from build123d import *

# Parameters (mm, degrees)
SKETCH1_R           = 20
BOSS_EXTRUDE1_DEPTH = 2
CUT_EXTRUDE10_DEPTH = 29.354893758
CIRPATTERN1_DEPTH   = 2
SKETCH5_R           = 0.76
CUT_EXTRUDE11_DEPTH = 28.141520821
SCALE1_SCALE        = 1.5
SCALE2_SCALE        = 0.93


# Read off the part's stored shape, not the designer's step: CirPattern1
with BuildPart() as part:
    # Sketch1 → Boss-Extrude1 (new body)
    with BuildSketch(Plane(origin=(0, 0, 0), x_dir=(1, 0, 0), z_dir=(0, 1, 0))):
        with Locations(Location((0, 0, 0), (0, 0, 270))):
            Circle(SKETCH1_R)
    extrude(amount=BOSS_EXTRUDE1_DEPTH)

    # Sketch3 → Cut-Extrude10 (cut, through all)
    with BuildSketch(Plane(origin=(0, 2, 0), x_dir=(1, 0, 0), z_dir=(0, 1, 0))):
        with BuildLine():
            Line((-0.11374729, 19.999676536), (2.525531299, 21.841438752))
            Line((2.525531299, 21.841438752), (8.448237607, 18.128079913))
            add(Edge.make_bspline(
                [(0.314716636, 11.921594207), (-1.061906761, 18.280624108), (8.448237607, 18.128079913)],
                knots=[0, 0, 0, 1, 1, 1], degree=2))
            add(Edge.make_bspline(
                [(-0.11374729, 19.999676536), (-3.476973379, 16.23883842), (0.314716636, 11.921594207)],
                knots=[0, 0, 0, 1, 1, 1], degree=2))
        make_face()
    extrude(amount=-CUT_EXTRUDE10_DEPTH, mode=Mode.SUBTRACT)

    # CirPattern1 outline → CirPattern1 (cut)
    with BuildSketch(Plane(origin=(0, 0, 0), x_dir=(1, 0, 0), z_dir=(0, 1, 0))):
        with BuildLine():
            add(Edge.make_bspline(
                [(-7.207557435, 17.244057808), (-7.782239787, 13.703261178), (-3.697405485, 11.367556407)],
                knots=[0.181076354, 0.181076354, 0.181076354, 1, 1, 1], degree=2))
            add(Edge.make_bspline(
                [(-3.697405485, 11.367556407), (-6.402099222, 15.840148745), (-1.097148713, 18.619435028)],
                knots=[0, 0, 0, 0.803340706, 0.803340706, 0.803340706], degree=2))
            add(Edge.make_bspline(
                [(-0.11374729, 19.999676536), (-0.722748007, 19.318677683), (-1.097148713, 18.619435028)],
                knots=[0, 0, 0, 0.181076354, 0.181076354, 0.181076354], degree=2))
            ThreePointArc((-0.11374729, 19.999676536), (-4.271024547, -19.538637345), (8.448237607, 18.128079913))
            add(Edge.make_bspline(
                [(5.128765463, 17.936244047), (6.577979327, 18.158079147), (8.448237607, 18.128079913)],
                knots=[0.803340706, 0.803340706, 0.803340706, 1, 1, 1], degree=2))
            add(Edge.make_bspline(
                [(5.128765463, 17.936244047), (2.500458036, 15.495035196), (4.289346694, 11.142878787)],
                knots=[0.181076354, 0.181076354, 0.181076354, 1, 1, 1], degree=2))
            add(Edge.make_bspline(
                [(4.289346694, 11.142878787), (4.902086374, 16.33363986), (10.795510687, 15.268519209)],
                knots=[0, 0, 0, 0.803340706, 0.803340706, 0.803340706], degree=2))
            add(Edge.make_bspline(
                [(10.795510687, 15.268519209), (7.516952988, 13.812991814), (7.795771849, 9.115796046)],
                knots=[0.181076354, 0.181076354, 0.181076354, 1, 1, 1], degree=2))
            add(Edge.make_bspline(
                [(7.795771849, 9.115796046), (10.060748967, 13.826351118), (15.289007186, 10.905349896)],
                knots=[0, 0, 0, 0.803340706, 0.803340706, 0.803340706], degree=2))
            add(Edge.make_bspline(
                [(15.289007186, 10.905349896), (11.715481814, 10.593232934), (10.454016527, 6.060011853)],
                knots=[0.181076354, 0.181076354, 0.181076354, 1, 1, 1], degree=2))
            add(Edge.make_bspline(
                [(10.454016527, 6.060011853), (14.125785669, 9.779899189), (18.12231489, 5.319553202)],
                knots=[0, 0, 0, 0.803340706, 0.803340706, 0.803340706], degree=2))
            add(Edge.make_bspline(
                [(18.12231489, 5.319553202), (14.641068768, 6.18466939), (11.97601867, 2.306667841)],
                knots=[0.181076354, 0.181076354, 0.181076354, 1, 1, 1], degree=2))
            add(Edge.make_bspline(
                [(11.97601867, 2.306667841), (16.656686676, 4.632779929), (18.988400946, -0.883563127)],
                knots=[0, 0, 0, 0.803340706, 0.803340706, 0.803340706], degree=2))
            add(Edge.make_bspline(
                [(18.988400946, -0.883563127), (15.976681108, 1.065037449), (12.196845731, -1.737502929)],
                knots=[0.181076354, 0.181076354, 0.181076354, 1, 1, 1], degree=2))
            add(Edge.make_bspline(
                [(12.196845731, -1.737502929), (17.379189594, -1.057236426), (17.793411491, -7.031795185)],
                knots=[0, 0, 0, 0.803340706, 0.803340706, 0.803340706], degree=2))
            add(Edge.make_bspline(
                [(17.793411491, -7.031795185), (15.577584513, -4.210871331), (11.09256767, -5.6342518)],
                knots=[0.181076354, 0.181076354, 0.181076354, 1, 1, 1], degree=2))
            add(Edge.make_bspline(
                [(11.09256767, -5.6342518), (16.215000021, -6.673548315), (14.666842175, -12.458886631)],
                knots=[0, 0, 0, 0.803340706, 0.803340706, 0.803340706], degree=2))
            add(Edge.make_bspline(
                [(14.666842175, -12.458886631), (13.487027293, -9.071330369), (8.782850151, -8.961305569)],
                knots=[0.181076354, 0.181076354, 0.181076354, 1, 1, 1], degree=2))
            add(Edge.make_bspline(
                [(8.782850151, -8.961305569), (13.29027596, -11.607541197), (9.947505297, -16.576727895)],
                knots=[0, 0, 0, 0.803340706, 0.803340706, 0.803340706], degree=2))
            add(Edge.make_bspline(
                [(9.947505297, -16.576727895), (9.93155376, -12.989633509), (5.517986904, -11.358126335)],
                knots=[0.181076354, 0.181076354, 0.181076354, 1, 1, 1], degree=2))
            add(Edge.make_bspline(
                [(5.517986904, -11.358126335), (8.921956647, -15.324540386), (4.146814235, -18.939086981)],
                knots=[0, 0, 0, 0.803340706, 0.803340706, 0.803340706], degree=2))
            add(Edge.make_bspline(
                [(4.146814235, -18.939086981), (5.296454639, -15.541171808), (1.651776524, -12.564981378)],
                knots=[0.181076354, 0.181076354, 0.181076354, 1, 1, 1], degree=2))
            add(Edge.make_bspline(
                [(1.651776524, -12.564981378), (3.58341726, -17.421751343), (-2.106636126, -19.289965628)],
                knots=[0, 0, 0, 0.803340706, 0.803340706, 0.803340706], degree=2))
            add(Edge.make_bspline(
                [(-2.106636126, -19.289965628), (0.084014843, -16.4494465), (-2.396817106, -12.451089227)],
                knots=[0.181076354, 0.181076354, 0.181076354, 1, 1, 1], degree=2))
            add(Edge.make_bspline(
                [(-2.396817106, -12.451089227), (-2.146828623, -17.671908721), (-8.135187408, -17.591340689)],
                knots=[0, 0, 0, 0.803340706, 0.803340706, 0.803340706], degree=2))
            add(Edge.make_bspline(
                [(-8.135187408, -17.591340689), (-5.140916898, -15.616031929), (-6.189066045, -11.028791865)],
                knots=[0.181076354, 0.181076354, 0.181076354, 1, 1, 1], degree=2))
            add(Edge.make_bspline(
                [(-6.189066045, -11.028791865), (-7.647819946, -16.047904086), (-13.285552537, -14.027284533)],
                knots=[0, 0, 0, 0.803340706, 0.803340706, 0.803340706], degree=2))
            add(Edge.make_bspline(
                [(-13.285552537, -14.027284533), (-9.812138156, -13.131241495), (-9.314021278, -8.452217279)],
                knots=[0.181076354, 0.181076354, 0.181076354, 1, 1, 1], degree=2))
            add(Edge.make_bspline(
                [(-9.314021278, -8.452217279), (-12.323438943, -12.725723538), (-16.999609535, -8.984017946)],
                knots=[0, 0, 0, 0.803340706, 0.803340706, 0.803340706], degree=2))
            add(Edge.make_bspline(
                [(-16.999609535, -8.984017946), (-13.423449627, -9.264340798), (-11.433045416, -5.000577306)],
                knots=[0.181076354, 0.181076354, 0.181076354, 1, 1, 1], degree=2))
            add(Edge.make_bspline(
                [(-11.433045416, -5.000577306), (-15.667009745, -8.06537689), (-18.874882696, -3.008057118)],
                knots=[0, 0, 0, 0.803340706, 0.803340706, 0.803340706], degree=2))
            add(Edge.make_bspline(
                [(-18.874882696, -3.008057118), (-15.583509678, -4.434368529), (-12.316509314, -1.047910694)],
                knots=[0.181076354, 0.181076354, 0.181076354, 1, 1, 1], degree=2))
            add(Edge.make_bspline(
                [(-12.316509314, -1.047910694), (-17.316204575, -2.571885013), (-18.708157077, 3.253009868)],
                knots=[0, 0, 0, 0.803340706, 0.803340706, 0.803340706], degree=2))
            add(Edge.make_bspline(
                [(-18.708157077, 3.253009868), (-16.058242285, 0.835272872), (-11.868675951, 2.977449797)],
                knots=[0.181076354, 0.181076354, 0.181076354, 1, 1, 1], degree=2))
            add(Edge.make_bspline(
                [(-11.868675951, 2.977449797), (-17.092307584, 3.159447008), (-16.517499984, 9.120699256)],
                knots=[0, 0, 0, 0.803340706, 0.803340706, 0.803340706], degree=2))
            add(Edge.make_bspline(
                [(-16.517499984, 9.120699256), (-14.796202804, 5.973535993), (-10.13807502, 6.639293898)],
                knots=[0.181076354, 0.181076354, 0.181076354, 1, 1, 1], degree=2))
            add(Edge.make_bspline(
                [(-10.13807502, 6.639293898), (-15.019581485, 8.507540416), (-12.540303105, 13.959155852)],
                knots=[0, 0, 0, 0.803340706, 0.803340706, 0.803340706], degree=2))
            add(Edge.make_bspline(
                [(-12.540303105, 13.959155852), (-11.934152795, 10.423610295), (-7.312243985, 9.540803981)],
                knots=[0.181076354, 0.181076354, 0.181076354, 1, 1, 1], degree=2))
            add(Edge.make_bspline(
                [(-7.312243985, 9.540803981), (-11.322638312, 12.892846308), (-7.207557435, 17.244057808)],
                knots=[0, 0, 0, 0.803340706, 0.803340706, 0.803340706], degree=2))
        make_face()
    extrude(amount=CIRPATTERN1_DEPTH, mode=Mode.SUBTRACT)

    # Sketch5 → Cut-Extrude11 (cut, through all)
    with BuildSketch(Plane(origin=(0, 2, 0), x_dir=(1, 0, 0), z_dir=(0, 1, 0))):
        with Locations(Location((0, 0, 0), (0, 0, 270))):
            Circle(SKETCH5_R)
    extrude(amount=-CUT_EXTRUDE11_DEPTH, mode=Mode.SUBTRACT)


with BuildPart() as part_1:
    # Scale1: scaled about (-0.031329983, 0.999999987, 0.377918145)
    add(part.part.scale(SCALE1_SCALE).moved(Location((0.015664991, -0.499999994, -0.188959072))))


with BuildPart() as part_2:
    # Scale2: scaled about (-0.031329983, 0.999999987, 0.377918146)
    add(part_1.part.scale(SCALE2_SCALE).moved(Location((-0.002193099, 0.069999999, 0.02645427))))


solid = part_2.part
Geometry check sheet. Reference: the model listing, model coordinates, mm. Give positions to 0.01 mm unless a question says otherwise; leave off trailing zeros. One line per question, with ' | ' between items.
1. Scan lines: line 1 along Z through (x, y) = (22, 1.4); line 2 along Z through (x, y) = (-22.5, 2.3); line 3 along Z through (x, y) = (16.5, 1.05). Record each from-to range of solid material in increasing order. Write a range as from..to.
Ans:
line 1: -10.27..-7.6, -4.05..0.03, 3.16..7.51 | line 2: -12.04..-7.79, -2.96..1.11, 4.54..7.88, 12.38..13.26 | line 3: -16.92..-12.69, -10.13..7.42, 7.96..13.11
2. Cross-section at A-A (z = -20.5). Count the separate pieces of the cut face and the enclosed holes in it, plus the area to 3 significant figures.
Ans:
separate pieces: 4 | enclosed holes: 0 | area: 47.9 mm2
3. Gauge pin test, flat ends, axial feed: pin 1 (1 mm diameter, centred on y = 1, z = 12, fed in from +X); pin 2 (1.5 mm diameter, centred on y = 1.5, z = 13.5, fed in from -X). Record the tip position at first contact, or that the pin passes through.
Ans:
pin 1: x = 20.86 | pin 2: x = -23.23
4. Mould release check, pull along Z, two halves, no side actions. Record for faces 1 (the face through (0, -0.395, 6)), 2 (the face through (0.331, 1.02, 0.862)): released by +Z, released by -Z, zero draft, split by the parting line, or undercut.
Ans:
face 1: zero draft | face 2: undercut
